from build123d import *

# Parameters (mm, degrees)
F0_W     = 137.5
F0_H     = 35
F1_DEPTH = 2
F2_R     = 1.5
F3_DEPTH = 25
F4_SIZE  = 1.87


with BuildPart() as f1:
    # F0 (on Front) → F1 (new body)
    with BuildSketch(Plane.XZ):
        Rectangle(F0_W, F0_H)
    extrude(amount=F1_DEPTH)

    # F2 (on face) → F3 (cut)
    with BuildSketch(Plane(origin=(0, 0, 0), x_dir=(-1, 0, 0), z_dir=(0, 1, 0))):
        with Locations((-50, 0)):
            Circle(F2_R)
        with Locations((50, 0)):
            Circle(F2_R)
    extrude(amount=-F3_DEPTH, mode=Mode.SUBTRACT)

    # F4
    f4_edges = [f1.edges().sort_by_distance(p)[0] for p in [
        (51.5, -2, 0),
        (-48.5, -2, 0),
    ]]
    chamfer(f4_edges, length=F4_SIZE)


solid = f1.part
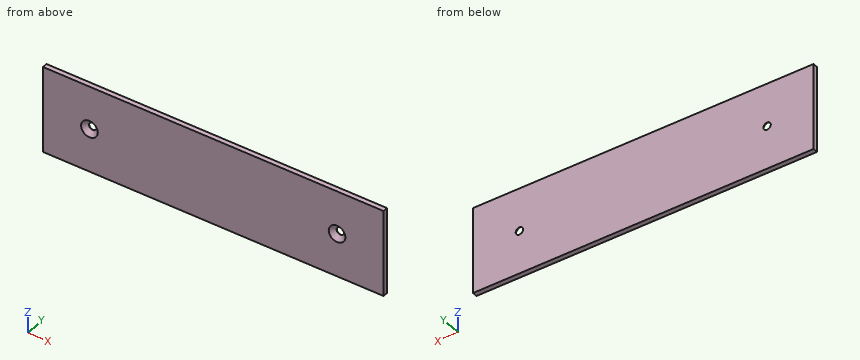
Verification items for the finished model (mm, model axes). Give positions to 0.01 mm unless a question says otherwise; leave off trailing zeros. Loops run counter-clockwise (first coordinate to the right, second up) from the corner with the lowest first, then second, coordinate; pieces in that order, holes last.
1. Material ranges on probe 1 along X at (y, z) = (-1.15, -0.5); probe 2 along X at (y, z) = (-1.25, 2), recorded low to high.
Derived:
probe 1: x = -68.75 to -52.47, -47.53 to 47.53, 52.47 to 68.75
probe 2: x = -68.75 to -51.69, -48.31 to 48.31, 51.69 to 68.75
2. Go/stop test with a flat-tipped pin: P1, Ø1.8, axis at x = 50, z = 0, coming from the +Y side. Record where the tip stops, or that it passes through.
Derived:
P1: passes through
3. Cross-section at B-B on z = 0. Record the cut outline in (x, y), and give its area (3 significant figures).
Derived:
outline: (-68.75, -2) - (-53.37, -2) - (-51.5, -0.13) - (-51.5, 0) - (-68.75, 0) - close; (-48.5, -0.13) - (-46.63, -2) - (46.63, -2) - (48.5, -0.13) - (48.5, 0) - (-48.5, 0) - close; (51.5, -0.13) - (53.37, -2) - (68.75, -2) - (68.75, 0) - (51.5, 0) - close
area: 256 mm2
4. Cross-section at A-A on x = -50. Record the cut outline in (y, z), and give its area (3 significant figures).
Derived:
outline: (-2, -17.5) - (0, -17.5) - (0, -1.5) - (-0.13, -1.5) - (-2, -3.37) - close; (-2, 3.37) - (-0.13, 1.5) - (0, 1.5) - (0, 17.5) - (-2, 17.5) - close
area: 60.5 mm2
